Design review of the part built by this model. Coordinates are the model's own, in mm. Coordinates: 2 decimals unless noted, no trailing zeros. Loops run counter-clockwise (first coordinate to the right, second up) from the corner with the lowest first, then second, coordinate; pieces in that order, holes last. Notation, with made-up numbers: M 5,-3.5 L 9,-3.5 A16 ccw 9,5.5 Z; hole C 66.25,38 d1. An arc over 180 degrees is marked long. One line per item, written item: value.
```python
from build123d import *

# Parameters (mm, degrees)
BOSS_EXTRUDE1_DEPTH = 3
BOSS_EXTRUDE2_DEPTH = 3
SKETCH6_R           = 2.5
CUT_EXTRUDE1_DEPTH  = 137.449762455
SKETCH7_W           = 20
SKETCH7_H           = 3
CUT_EXTRUDE2_DEPTH  = 137.449762455


with BuildPart() as part:
    # Sketch4 → Boss-Extrude1 (new body)
    with BuildSketch(Plane(origin=(0, 0, 0), x_dir=(1, 0, 0), z_dir=(0, 1, 0))):
        Polygon((-32.886751346, 91.602540378), (32.886751346, 91.602540378), (95.773502692, -17.320508076), (62.886751346, -74.282032303), (-62.886751346, -74.282032303), (-95.773502692, -17.320508076), align=None)
    extrude(amount=-BOSS_EXTRUDE1_DEPTH)

    # Sketch5 → Boss-Extrude2 (add, through all)
    with BuildSketch(Plane(origin=(0, 0, 0), x_dir=(1, 0, 0), z_dir=(0, 1, 0))):
        Polygon((-95.773502692, -17.320508076), (-32.886751346, 91.602540378), (-36.350852961, 93.602540378), (-99.237604307, -15.320508076), align=None)
    extrude(amount=-BOSS_EXTRUDE2_DEPTH)

    # Sketch6 → Cut-Extrude1 (cut, through all)
    with BuildSketch(Plane(origin=(0, 0, 0), x_dir=(1, 0, 0), z_dir=(0, 1, 0))):
        with Locations(Location((-56.883974596, 38.038130468, 0), (0, 0, 270))):
            Circle(SKETCH6_R)
    extrude(amount=-CUT_EXTRUDE1_DEPTH, mode=Mode.SUBTRACT)

    # Sketch7 → Cut-Extrude2 (cut, through all)
    with BuildSketch(Plane(origin=(0, 0, 0), x_dir=(1, 0, 0), z_dir=(0, 1, 0))):
        with Locations((0, 88.102540378)):
            Rectangle(SKETCH7_W, SKETCH7_H)
        with Locations((-30, -70.782032303)):
            Rectangle(SKETCH7_W, SKETCH7_H)
        with Locations((30, -70.782032303)):
            Rectangle(SKETCH7_W, SKETCH7_H)
        Polygon((50, 51.961524227), (40, 69.282032303), (42.598076211, 70.782032303), (52.598076211, 53.461524227), align=None)
        Polygon((72.598076211, 18.820508076), (70, 17.320508076), (80, 0), (82.598076211, 1.5), align=None)
        Polygon((80, -34.641016151), (70, -51.961524227), (72.598076211, -53.461524227), (82.598076211, -36.141016151), align=None)
        Polygon((-70, -51.961524227), (-80, -34.641016151), (-82.598076211, -36.141016151), (-72.598076211, -53.461524227), align=None)
        Polygon((-45.196152423, 72.282032303), (-55.196152423, 54.961524227), (-52.598076211, 53.461524227), (-42.598076211, 70.782032303), align=None)
        Polygon((-75.196152423, 20.320508076), (-85.196152423, 3), (-82.598076211, 1.5), (-72.598076211, 18.820508076), align=None)
    extrude(amount=-CUT_EXTRUDE2_DEPTH, mode=Mode.SUBTRACT)


solid = part.part
```
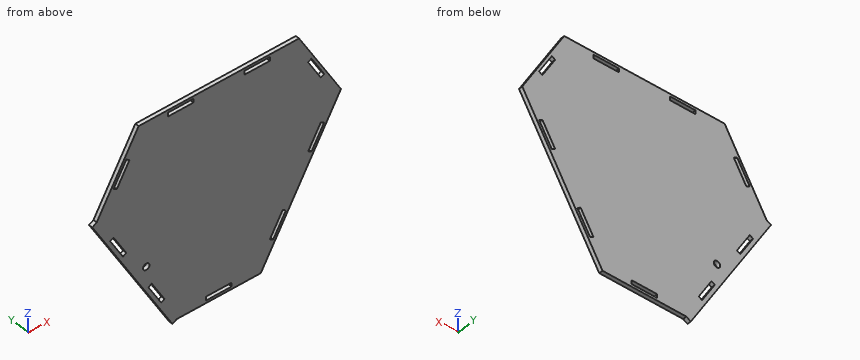
(1) We need section B-B on y = -2. State how many separate pieces and enclosed holes the cut face has, then the cut area to 3 significant figures.
Reply:
separate pieces: 1
enclosed holes: 10
area: 23,000 mm2
(2) We need section A-A on z = -9.5. State the section outline as (x, y) points.
Reply:
outline: M -84.91,-3 L -81.44,-3 L -81.44,0 L -84.91,0 Z; M -77.98,-3 L 74.52,-3 L 74.52,0 L -77.98,0 Z; M 77.98,-3 L 80.29,-3 L 80.29,0 L 77.98,0 Z
(3) We need section C-C on z = 32. State the section outline as (x, y) points, then the cut area to 3 significant figures.
Reply:
outline: M -87.3,-3 L 87.3,-3 L 87.3,0 L -87.3,0 Z
area: 524 mm2
(4) We need section D-D on z = -76. State the section outline as (x, y) points.
Reply:
outline: M -46.51,-3 L 41.89,-3 L 41.89,0 L -46.51,0 Z
(5) To check wall thickness, follow line 1 along Z through (x, y) = (28.5, -1.3); line 2 along X through (y, z) = (-2.05, 47); line 3 along X through (y, z) = (-0.25, -18). State the ranges of each line that lie inside material, in increasing order. Write a range as [from, to].
Reply:
line 1: z = [-91.6, 69.28], [72.28, 74.28]
line 2: x = [-78.64, -76.33], [-72.86, 72.86], [76.33, 78.64]
line 3: x = [-80, -76.54], [-73.07, 71.18], [73.07, 75.38]
(6) Insertion check: pin 1 (0.9 mm diameter, centred on y = -1, z = -88, fed in from +X); pin 2 (1 mm diameter, centred on x = 20.5, y = -2.5, fed in from -Z); pin 3 (1.5 mm diameter, centred on y = -1, z = -87.5, fed in from -X). Each pin has a flat end and moves straight along its axis. Give the tip position at first contact, or say it passes through.
Reply:
pin 1: stops at x = 35.23
pin 2: stops at z = -91.6
pin 3: stops at x = -40.31
